Could you check a few things on this model? Use its own coordinates, in mm. Face numbers are marked on the shaded views. A direction names the side the tool comes from. Round coordinates to 2 decimals unless told otherwise and drop trailing zeros. Write each loop counter-clockwise with the first axis right and the second up, starting at its lowest first coordinate (ties: lowest second). Pieces come first, ordered by that corner, then holes. Notation, with made-up numbers: M 3.25,70.25 L 24.25,70.25 A15 cw 24.25,86.25 Z; hole C 87.5,70.25 d1. An arc over 180 degrees is marked long. One line per item, written item: value. Start each with the question number.
(1) I'm going to push flat-ended pins straight in: pin 1 Ø7.5 at (y, z) = (42, -21.5) entering from +X; pin 2 Ø10.5 at (y, z) = (-43.5, -15.5) entering from -X; pin 3 Ø5.5 at (x, y) = (30.75, -30.75) entering from -Z. Where does each tip first touch, or does it pass through?
(2) If I drill on L1, parallel to Z at x = 6, y = -49.1; L2, parallel to Y at x = -30, z = 1; L3, parallel to Y at x = -30.75, z = 3.25, over which ranges is the centre line in solid material (lowest first)?
(3) I want a section at C-C on x = -11.5. Please give me the cut outline in (y, z), and give its area (3 significant figures).
(4) I want a section at A-A on z = -51. Please give me the cut outline in (x, y).
(5) I want a section at D-D on x = 6. Please give me the cut outline in (y, z).
(6) I want a section at B-B on z = -69. Please give me the cut outline in (x, y).
(7) Which directions (+Z, -Z, +X, -X, +Y, -Y) give clear straight access to the entire face, cutting with the end or side of a thin tool? Please do the marked faces 1 and 2.
```python
from build123d import *

# Parameters (mm, degrees)
F0_R     = 1.75
F0_R_2   = 35
F1_DEPTH = 5
F2_W     = 10
F2_H     = 5
F3_DEPTH = 74
F4_R     = 2.25
F5_DEPTH = 102.001


with BuildPart() as f1:
    # F0 (on Top) → F1 (new body)
    with BuildSketch(Plane.XY):
        with BuildLine():
            Line((-24.280967, 29.230714), (-28.275126, 33.224874))
            ThreePointArc((-28.275126, 33.224874), (-33.224874, 33.224874), (-33.224874, 28.275126))
            Line((-33.224874, 28.275126), (-29.230714, 24.280967))
            ThreePointArc((-29.230714, 24.280967), (-35.740503, 12.907999), (-38, 0))
            ThreePointArc((-38, 0), (-35.740503, -12.907999), (-29.230714, -24.280967))
            Line((-29.230714, -24.280967), (-33.224874, -28.275126))
            ThreePointArc((-33.224874, -28.275126), (-33.224874, -33.224874), (-28.275126, -33.224874))
            Line((-28.275126, -33.224874), (-24.280967, -29.230714))
            ThreePointArc((-24.280967, -29.230714), (-12.907999, -35.740503), (0, -38))
            ThreePointArc((0, -38), (0.500043, -37.99671), (1, -37.98684))
            ThreePointArc((1, -37.98684), (6.054012, -37.51465), (11, -36.373067))
            ThreePointArc((11, -36.373067), (17.998332, -33.467298), (24.280967, -29.230714))
            Line((24.280967, -29.230714), (28.275126, -33.224874))
            ThreePointArc((28.275126, -33.224874), (33.224874, -33.224874), (33.224874, -28.275126))
            Line((33.224874, -28.275126), (29.230714, -24.280967))
            ThreePointArc((29.230714, -24.280967), (35.740503, -12.907999), (38, 0))
            ThreePointArc((38, 0), (35.740503, 12.907999), (29.230714, 24.280967))
            Line((29.230714, 24.280967), (33.224874, 28.275126))
            ThreePointArc((33.224874, 28.275126), (33.224874, 33.224874), (28.275126, 33.224874))
            Line((28.275126, 33.224874), (24.280967, 29.230714))
            ThreePointArc((24.280967, 29.230714), (17.998332, 33.467298), (11, 36.373067))
            ThreePointArc((11, 36.373067), (6.054012, 37.51465), (1, 37.98684))
            ThreePointArc((1, 37.98684), (0.500043, 37.99671), (0, 38))
            ThreePointArc((0, 38), (-12.907999, 35.740503), (-24.280967, 29.230714))
        make_face()
        with Locations((-30.75, -30.75)):
            Circle(F0_R, mode=Mode.SUBTRACT)
        with Locations((30.75, -30.75)):
            Circle(F0_R, mode=Mode.SUBTRACT)
        with Locations((-30.75, 30.75)):
            Circle(F0_R, mode=Mode.SUBTRACT)
        Circle(F0_R_2, mode=Mode.SUBTRACT)
        with Locations((30.75, 30.75)):
            Circle(F0_R, mode=Mode.SUBTRACT)
        with BuildLine():
            Line((1, 51), (1, 37.98684))
            ThreePointArc((1, 37.98684), (6.054012, 37.51465), (11, 36.373067))
            Line((11, 36.373067), (11, 51))
            Line((11, 51), (1, 51))
        make_face()
        with BuildLine():
            ThreePointArc((11, -36.373067), (6.054012, -37.51465), (1, -37.98684))
            Line((1, -37.98684), (1, -51))
            Line((1, -51), (11, -51))
            Line((11, -51), (11, -36.373067))
        make_face()
    extrude(amount=F1_DEPTH)

    # F2 (on face) → F3 (join)
    with BuildSketch(Plane(origin=(0, 0, 0), x_dir=(1, 0, 0), z_dir=(0, 0, -1))):
        with Locations((6, -48.5)):
            Rectangle(F2_W, F2_H)
        with Locations((6, 48.5)):
            Rectangle(F2_W, F2_H)
    extrude(amount=F3_DEPTH)

    # F4 (on face) → F5 (cut, through all)
    with BuildSketch(Plane(origin=(0, 51, 0), x_dir=(-1, 0, 0), z_dir=(0, 1, 0))):
        with Locations((-6, -69)):
            Circle(F4_R)
        with Locations((-6, -45)):
            Circle(F4_R)
    extrude(amount=-F5_DEPTH, mode=Mode.SUBTRACT)


solid = f1.part
```
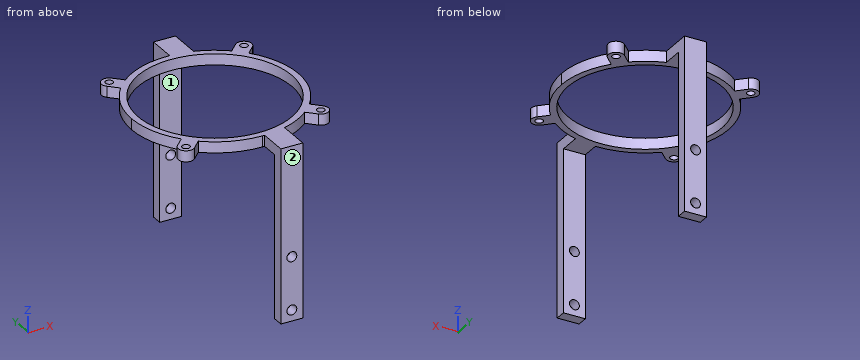
Found:
1. pin 1: passes through
1. pin 2: stops at x = 1
1. pin 3: stops at z = 0
2. L1: z = -74 to -71.25, -66.75 to -47.25, -42.75 to 5
2. L2: y = -34.17 to -32.33, -29.17 to -25.05, -23.32 to -18.03, 18.03 to 23.32, 25.05 to 29.17, 32.33 to 34.17
2. L3: y = -34.25 to -32.5, -29 to -25.8, -22.33 to -16.72, 16.72 to 22.33, 25.8 to 29, 32.5 to 34.25
3. outline: M -36.22,0 L -33.06,0 L -33.06,5 L -36.22,5 Z; M 33.06,0 L 36.22,0 L 36.22,5 L 33.06,5 Z
3. area: 31.6 mm²
4. outline: M 1,-51 L 11,-51 L 11,-46 L 1,-46 Z; M 1,46 L 11,46 L 11,51 L 1,51 Z
5. outline: M -51,-74 L -46,-74 L -46,-71.25 L -51,-71.25 Z; M -51,-66.75 L -46,-66.75 L -46,-47.25 L -51,-47.25 Z; M -51,-42.75 L -46,-42.75 L -46,0 L -34.48,0 L -34.48,5 L -51,5 Z; M 34.48,0 L 46,0 L 46,-42.75 L 51,-42.75 L 51,5 L 34.48,5 Z; M 46,-74 L 51,-74 L 51,-71.25 L 46,-71.25 Z; M 46,-66.75 L 51,-66.75 L 51,-47.25 L 46,-47.25 Z
6. outline: M 1,-51 L 3.75,-51 L 3.75,-46 L 1,-46 Z; M 1,46 L 3.75,46 L 3.75,51 L 1,51 Z; M 8.25,-51 L 11,-51 L 11,-46 L 8.25,-46 Z; M 8.25,46 L 11,46 L 11,51 L 8.25,51 Z
7. face 1: -Z, +X, -X
7. face 2: +Z, -Z, +X, -X, -Y
